Geometry check sheet. Reference: the model listing, model coordinates, mm. Round coordinates to 2 decimals unless told otherwise and drop trailing zeros. Write each loop counter-clockwise with the first axis right and the second up, starting at its lowest first coordinate (ties: lowest second). Pieces come first, ordered by that corner, then holes. Notation, with made-up numbers: (-1.75, 27.25) -> (24.25, 27.25) arc R13 cw to (24.25, 44.25) -> close; hole circle Ø10 at (51.5, 50.25). An arc over 180 degrees is marked (long way). One line per question, with ' | ' between items.
Autodesk Inventor part; units mm, degrees
ref_plane "YZ Plane" through (0, 0, 0) normal (1, 0, 0) x (0, 1, 0)
ref_plane "XZ Plane" through (0, 0, 0) normal (0, 1, 0) x (-1, 0, 0)
ref_plane "XY Plane" through (0, 0, 0) normal (0, 0, 1) x (1, 0, 0)
sketch "Sketch1" plane through (0, 0, 0) normal (0, 1, 0) x (-1, 0, 0)
  line L0 (-107, 107) -> (107, 107)
  line L1 (107, 107) -> (107, -107)
  line L2 (107, -107) -> (-107, -107)
  line L3 (-107, -107) -> (-107, 107)
  line L4 (-107, 107) -> (107, -107) construction
  line L5 (107, 107) -> (-107, -107) construction
  point P0 (0, 0)
  dimension "d0" = 214
  dimension "d1" = 214
extrude "Extrusion1" add sketch "Sketch1" along normal blind 1.6
sketch "Sketch2" plane through (0, 1.6, 0) normal (0, 1, 0) x (1, 0, 0)
  line L0 (-107, 107) -> (-107, -107)
  line L1 (0, 13.9914) -> (-10, -3.3291)
  line L2 (0, 13.9914) -> (20, 13.9914) construction
  line L3 (-10, -3.3291) -> (10, -3.3291)
  line L4 (10, -3.3291) -> (0, 13.9914)
  line L5 (-5.4032, 2.7326) -> (4.9323, 2.7326) construction
  line L6 (4.9323, 2.7326) -> (4.9323, -0.9149) construction
  line L7 (4.9323, -0.9149) -> (-5.4032, -0.9149) construction
  line L8 (-5.4032, -0.9149) -> (-5.4032, 2.7326) construction
  line L9 (0.0715, 16.0255) -> (-12.0985, -5.0535)
  line L10 (-12.0985, -5.0535) -> (12.2415, -5.0535)
  line L11 (12.2415, -5.0535) -> (0.0715, 16.0255)
  point P0 (0, 0)
  dimension "d4" = 20
  dimension "d6" = 20
  dimension "d9" = 24.34
  dimension "d10" = 24.34
extrude "Extrusion2" add sketch "Sketch2" along normal blind 0.1
sketch "Sketch3" plane through (0, 1.6, 0) normal (0, 1, 0) x (1, 0, 0)
  line L0 (104.5, -104.5) -> (-104.5, 104.5) construction
  circle A0 centre (-104.5, 104.5) radius 1.5
  circle A1 centre (104.5, 104.5) radius 1.5
  circle A2 centre (104.5, -104.5) radius 1.5
  circle A3 centre (-104.5, -104.5) radius 1.5
  point P0 (0, 0)
  dimension "d15" = 3
  dimension "d16" = 3
  dimension "d17" = 3
  dimension "d18" = 3
extrude "Extrusion3" cut sketch "Sketch3" against normal blind 10
properties part number "Heatbed" material "Aluminum, Anodized Red"
(1) Material ranges on line 1 (X direction, y = 0.85, z = 104.5); line 2 (Y direction, x = -29, z = -1), recorded low to high.
Resolved:
line 1: x = -107 to -106, -103 to 103, 106 to 107 | line 2: y = 0 to 1.6
(2) Sectioned sample at C-C on x = -67. Record the cut outline in (y, z).
Resolved:
outline: (0, -107) -> (1.6, -107) -> (1.6, 107) -> (0, 107) -> close
(3) Sectioned sample at A-A on x = -2.5. Record the cut outline in (y, z).
Resolved:
outline: (0, -107) -> (1.6, -107) -> (1.6, -11.57) -> (1.7, -11.57) -> (1.7, -9.66) -> (1.6, -9.66) -> (1.6, 3.33) -> (1.7, 3.33) -> (1.7, 5.05) -> (1.6, 5.05) -> (1.6, 107) -> (0, 107) -> close
(4) Sectioned sample at B-B on z = 17. Record the cut outline in (x, y), then the cut area to 3 significant figures.
Resolved:
outline: (-107, 0) -> (107, 0) -> (107, 1.6) -> (-107, 1.6) -> close | area: 342 mm2
(5) Go/stop test with a flat-tipped pin: pin 1 (5 mm diameter, centred on x = -104.5, z = -104.5, fed in from +Y). Record where the tip stops, or that it passes through.
Resolved:
pin 1: stops at y = 1.6
